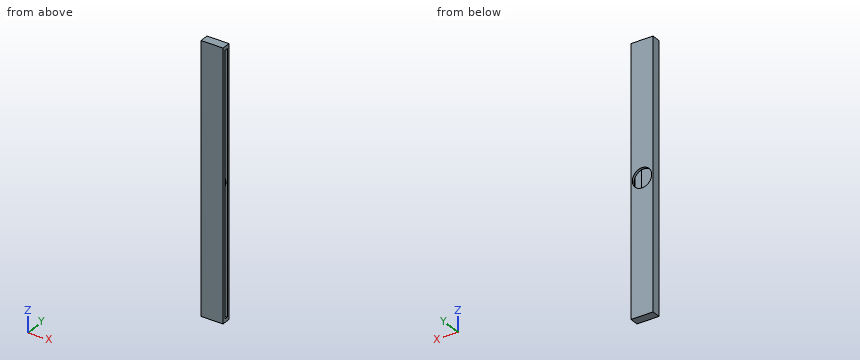
```python
from build123d import *

# Parameters (mm, degrees)
SKETCH_1_W          = 15
SKETCH_1_H          = 300
EXTRUDE_1_DEPTH     = 4
SKETCH_2_W          = 4
SKETCH_2_H          = 4
EXTRUDE_2_DEPTH     = 10
SKETCH_3_W          = 25
SKETCH_3_H          = 300
EXTRUDE_3_DEPTH     = 3
SKETCH_4_W          = 25
SKETCH_4_H          = 300
EXTRUDE_4_DEPTH     = 3
SKETCH_5_R          = 11
CUT_EXTRUDE_1_DEPTH = 3


with BuildPart() as part:
    # 草图1 → 凸台-拉伸1 (new body)
    with BuildSketch(Plane(origin=(0, 0, 0), x_dir=(1, 0, 0), z_dir=(0, 1, 0))):
        with Locations((-54.836215811, -65.70889057)):
            Rectangle(SKETCH_1_W, SKETCH_1_H)
    extrude(amount=EXTRUDE_1_DEPTH)

    # 草图2 → 凸台-拉伸2 (add)
    with BuildSketch(Plane(origin=(-47.336215811, 0, 0), x_dir=(0, 0, -1), z_dir=(1, 0, 0))):
        with Locations((-213.70889057, 2)):
            Rectangle(SKETCH_2_W, SKETCH_2_H)
        with Locations((82.29110943, 2)):
            Rectangle(SKETCH_2_W, SKETCH_2_H)
    extrude(amount=EXTRUDE_2_DEPTH)

    # 草图3 → 凸台-拉伸3 (add)
    with BuildSketch(Plane(origin=(0, 4, 0), x_dir=(1, 0, 0), z_dir=(0, 1, 0))):
        with Locations((-49.836215811, -65.70889057)):
            Rectangle(SKETCH_3_W, SKETCH_3_H)
    extrude(amount=EXTRUDE_3_DEPTH)

    # 草图4 → 凸台-拉伸4 (add)
    with BuildSketch(Plane.XZ):
        with Locations((-49.836215811, 65.70889057)):
            Rectangle(SKETCH_4_W, SKETCH_4_H)
    extrude(amount=EXTRUDE_4_DEPTH)

    # 草图5 → 切除-拉伸1 (cut)
    with BuildSketch(Plane(origin=(0, 7, 0), x_dir=(1, 0, 0), z_dir=(0, 1, 0))):
        with Locations(Location((-49.836215811, -65.70889057, 0), (0, 0, 270))):
            Circle(SKETCH_5_R)
    extrude(amount=-CUT_EXTRUDE_1_DEPTH, mode=Mode.SUBTRACT)


solid = part.part
```
For this review, take the finished solid that the model builds, in its own axes (mm). Round coordinates to 2 decimals unless told otherwise and drop trailing zeros. Order: outer loops, then holes, each group sorted by start corner. A loop starts at its lowest first (then second) coordinate and runs counter-clockwise, first axis right, second up. Notation, with made-up numbers: (-16, 36.5) -> (6, 36.5) arc R25 ccw to (6, 64.5) -> close; hole circle Ø4 at (-37, -16.5). An arc over 180 degrees is marked (long way). Use a Markdown table: item, result.
Item 1: Take a section at B-B (z = -17). State the section outline as (x, y) points, plus the area to 3 significant figures.
Resolved:
| item | result |
|---|---|
| outline | (-62.34, -3) -> (-37.34, -3) -> (-37.34, 0) -> (-47.34, 0) -> (-47.34, 4) -> (-37.34, 4) -> (-37.34, 7) -> (-62.34, 7) -> close |
| area | 210 mm² |
Item 2: For pin 1 (2 mm diameter, centred on y = 2, z = 134.5, fed in from +X), flat-tipped, find the tip position at first contact; note if it passes through.
Resolved:
| item | result |
|---|---|
| pin 1 | stops at x = -47.34 |
Item 3: For line 1 along Y through (x, z) = (-40.75, 78); line 2 along Z through (x, y) = (-45.75, 2.75); line 3 along X through (y, z) = (3.75, 198), list the stretches that pass through material, from the lowest coordinate up. Write a range as [from, to].
Resolved:
| item | result |
|---|---|
| line 1 | y = [-3, 0], [4, 7] |
| line 2 | z = [-84.29, -80.29], [211.71, 215.71] |
| line 3 | x = [-62.34, -47.34] |
Item 4: Take a section at A-A (y = 1.5). State the section outline as (x, z) points.
Resolved:
| item | result |
|---|---|
| outline | (-62.34, -84.29) -> (-37.34, -84.29) -> (-37.34, -80.29) -> (-47.34, -80.29) -> (-47.34, 211.71) -> (-37.34, 211.71) -> (-37.34, 215.71) -> (-62.34, 215.71) -> close |
Item 5: Take a section at C-C (x = -42.25). State the section outline as (y, z) points, plus the area to 3 significant figures.
Resolved:
| item | result |
|---|---|
| outline | (-3, -84.29) -> (7, -84.29) -> (7, 57.74) -> (4, 57.74) -> (4, -80.29) -> (0, -80.29) -> (0, 211.71) -> (4, 211.71) -> (4, 73.67) -> (7, 73.67) -> (7, 215.71) -> (-3, 215.71) -> close |
| area | 1,780 mm² |
